For this review, use the dimensioned drawing (mm, ordinates from the lowest corner) and the shaded views. A direction names the side the tool comes from. Round coordinates to 2 decimals unless told otherwise and drop trailing zeros. Order: outer loops, then holes, each group sorted by start corner. A loop starts at its lowest first (then second) coordinate and runs counter-clockwise, first axis right, second up. Notation, with made-up numbers: (44, -15.75) - (98, -15.75) arc R12 cw to (98, -3.75) - close; hole circle Ø7 at (89.5, 22.5). An arc over 180 degrees is marked (long way). Use CSV: the item, a comma, the result in double quotes. Start each with the question number.
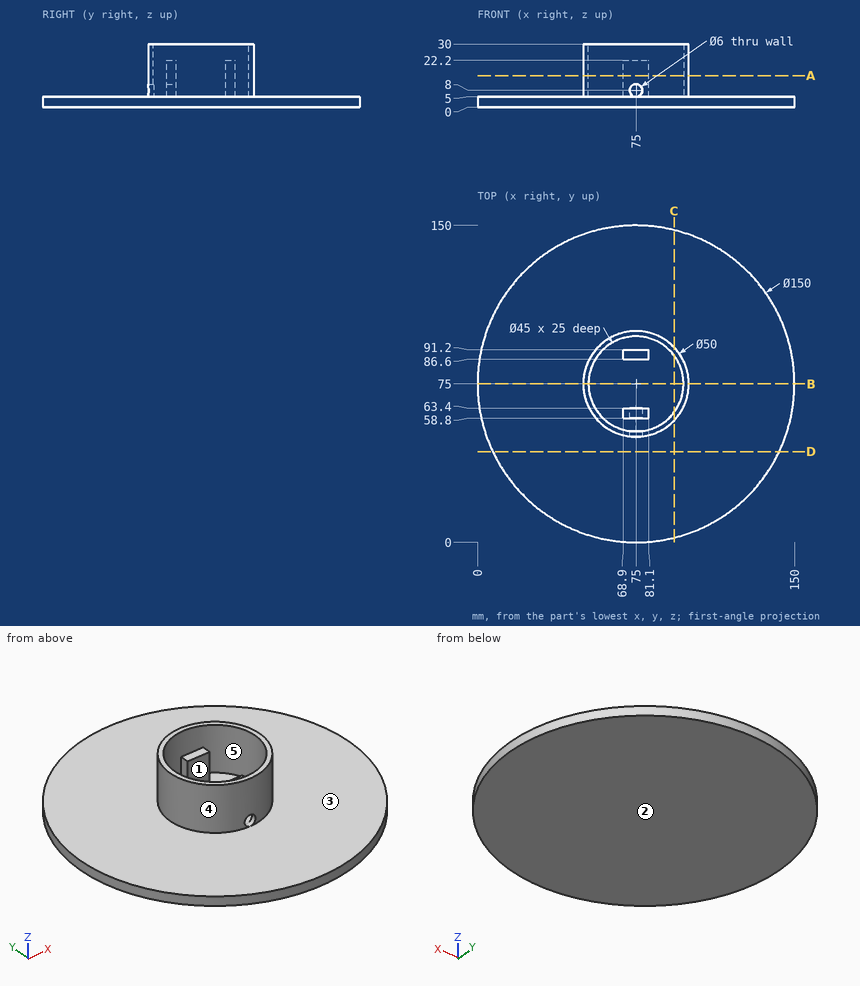
Q1. Take a section at B-B (y = 75). State the section outline as (x, z) points.
Q2. Tool access review of the marked faces 1 and 2: name each direction out of +Z, -Z, +X, -X, +Y, -Y from which nothing blocks a thin tool from reaching the whole face with its end or side.
Q3. For L1, parallel to Y at x = 75, z = 12; L2, parallel to X at y = 75, z = 20; L3, parallel to X at y = 62, z = 8, list the stretches that pass through material, from the lowest coordinate up. Write a range as [from, to].
Q4. The part is to be moulded in two halves that separate along X. For the marked faces 3, 4 and 5, say which applies: +X half, -X half, draft (parallel to the pull), parting line (faces both ways), or undercut.
Q5. Take a section at A-A (z = 15). State the section outline as (x, y) points, plus the area to 3 significant figures.
Q6. Take a section at C-C (x = 93). State the section outline as (y, z) points.
Q7. Clearance check with flat-ended pins moving along their axes: pin 1 (3.5 mm diameter, centred on y = 61, z = 12, fed in from +X); pin 2 (22.5 mm diameter, centred on x = 65.5, y = 71.5, fed in from +Z); pin 3 (6 mm diameter, centred on x = 72, z = 11, fed in from +Y). State where each tip first meets the part, or that it passes through.
Q8. Take a section at D-D (y = 43). State the section outline as (x, z) points, plus the area to 3 significant figures.
Findings below:
1,outline,"(0, 0) - (150, 0) - (150, 5) - (100, 5) - (100, 30) - (97.5, 30) - (97.5, 5) - (52.5, 5) - (52.5, 30) - (50, 30) - (50, 5) - (0, 5) - close"
2,face 1,"+Z"
2,face 2,"-Z, +X, -X, +Y, -Y"
3,L1,"y = [50, 52.5], [58.8, 63.4], [86.6, 91.2], [97.5, 100]"
3,L2,"x = [50, 52.5], [97.5, 100]"
3,L3,"x = [53.65, 56.64], [68.9, 72], [78, 81.1], [93.36, 96.35]"
4,face 3,"draft"
4,face 4,"parting line"
4,face 5,"undercut"
5,outline,"circle Ø50 at (75, 75); (68.9, 58.8) - (81.1, 58.8) - (81.1, 63.4) - (68.9, 63.4) - close; (68.9, 86.6) - (81.1, 86.6) - (81.1, 91.2) - (68.9, 91.2) - close; hole circle Ø45 at (75, 75)"
5,area,"485 mm^2"
6,outline,"(2.19, 0) - (147.81, 0) - (147.81, 5) - (92.35, 5) - (92.35, 30) - (88.5, 30) - (88.5, 5) - (61.5, 5) - (61.5, 30) - (57.65, 30) - (57.65, 5) - (2.19, 5) - close"
7,pin 1,"stops at x = 96.79"
7,pin 2,"stops at z = 22.2"
7,pin 3,"stops at y = 100"
8,outline,"(7.17, 0) - (142.83, 0) - (142.83, 5) - (7.17, 5) - close"
8,area,"678 mm^2"
